Read the model definition and answer for the solid it produces. Units are mm, in the model's axes. Face numbers are marked on the shaded views. A direction names the side the tool comes from. Coordinates: 2 decimals unless noted, no trailing zeros. Loops run counter-clockwise (first coordinate to the right, second up) from the corner with the lowest first, then second, coordinate; pieces in that order, holes last.
Q1. The mould has two halves that part along Z. Classify the marked faces 4, 5 and 6: pulls with the +Z half, pulls with the -Z half, needs draft (parallel to the pull), parting line crosses it, or undercut.
Q2. Which of the six approach directions +Z, -Z, +X, -X, +Y, -Y give full straight-line access (tool end or side, diameter ignored) to the marked faces 1, 2 and 3?
Q3. Flat-ended cylindrical pins translate along their axes: P1, Ø12.5, axis at x = 92, y = 260, coming from the -Z side; P2, Ø1.5, axis at x = -83, y = 126.5, coming from the -Z side; P3, Ø12.5, axis at x = -92, y = 127.5, coming from the +Z side. Find the tip coordinate at first contact, or state that the pin passes through.
Q4. Section B-B (x = 92) is taken. Count the separate pieces of the cut face and the enclosed holes in it, then the cut area to 3 significant figures.
Q5. Straight lines are drawn through the part: line 1 (X direction, y = 127, z = 3); line 2 (Y direction, x = 92, z = 1); line 3 (Z direction, x = 95.5, y = -28). For each, find the intervals that lie inside material, in ascending order.
Q6. Section A-A (y = 127.5) is taken. Give the vertices of the cut face in (x, z), then the cut area to 3 significant figures.
Q7. Section C-C (y = -160) is taken. Give the vertices of the cut face in (x, z).
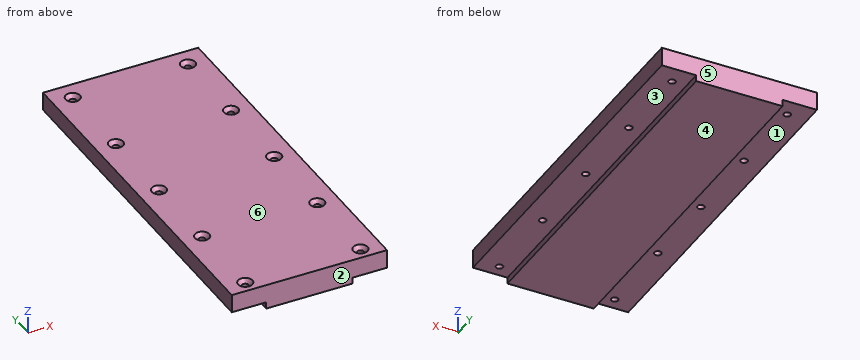
from build123d import *

# Parameters (mm, degrees)
SKETCH2_W                  = 580
SKETCH2_H                  = 248
BOSS_EXTRUDE1_DEPTH        = 20
SKETCH3_W                  = 55
SKETCH3_H                  = 10.706810323
SKETCH3_H_2                = 10
CUT_EXTRUDE1_DEPTH         = 594.444184402
F_11_0_11_DIAMETER_HOLE1_D = 11
LPATTERN1_COUNT            = 5
LPATTERN1_PITCH            = 132.5
CHAMFER1_SIZE              = 6


with BuildPart() as part:
    # Sketch2 → Boss-Extrude1 (new, symmetric)
    with BuildSketch(Plane(origin=(0, 0, 0), x_dir=(0, 1, 0), z_dir=(0, 0, 1))):
        Rectangle(SKETCH2_W, SKETCH2_H)
    extrude(amount=BOSS_EXTRUDE1_DEPTH, both=True)

    # Sketch3 → Cut-Extrude1 (cut, through all)
    with BuildSketch(Plane(origin=(0, 290, 0), x_dir=(-1, 0, 0), z_dir=(0, 1, 0))):
        with Locations((96.5, -14.646594839)):
            Rectangle(SKETCH3_W, SKETCH3_H)
        with Locations((-96.5, -15)):
            Rectangle(SKETCH3_W, SKETCH3_H_2)
    extrude(amount=-CUT_EXTRUDE1_DEPTH, mode=Mode.SUBTRACT)

    # Ø11.0 (11) Diameter Hole1 (through all)
    with Locations(Plane(origin=(-92, -270, 20), x_dir=(1, 0, 0), z_dir=(0, 0, 1))):
        with Locations((0, 0), (184, 0)):
            f_11_0_11_diameter_hole1 = Hole(F_11_0_11_DIAMETER_HOLE1_D / 2)

    # LPattern1: Ø11.0 (11) Diameter Hole1 ×5
    with Locations(*[(0, i * LPATTERN1_PITCH, 0) for i in range(1, LPATTERN1_COUNT)]):
        add(f_11_0_11_diameter_hole1, mode=Mode.SUBTRACT)

    # Chamfer1
    chamfer1_edges = [part.edges().sort_by_distance(p)[0] for p in [
        (97.5, -270, 20),
        (-86.5, -270, 20),
        (97.5, -137.5, 20),
        (-86.5, -137.5, 20),
        (97.5, -5, 20),
        (-86.5, -5, 20),
        (97.5, 127.5, 20),
        (-86.5, 127.5, 20),
        (97.5, 260, 20),
        (-86.5, 260, 20),
    ]]
    chamfer(chamfer1_edges, length=CHAMFER1_SIZE)


solid = part.part
Numbers:
1. face 4: pulls with the -Z half
1. face 5: needs draft
1. face 6: pulls with the +Z half
2. face 1: -Z, -X, +Y, -Y
2. face 2: +Z, -Z, +X, -X, -Y
2. face 3: -Z, +X, +Y, -Y
3. P1: stops at z = -10
3. P2: stops at z = -9.29
3. P3: stops at z = 14.75
4. separate pieces: 6
4. enclosed holes: 0
4. area: 15,600 mm2
5. line 1: x = -124 to -97.48, -86.52 to 86.52, 97.48 to 124
5. line 2: y = -290 to -275.5, -264.5 to -143, -132 to -10.5, 0.5 to 122, 133 to 254.5, 265.5 to 290
5. line 3: z = -10 to 20
6. outline: (-124, -9.29) - (-97.5, -9.29) - (-97.5, 14) - (-103.5, 20) - (-124, 20) - close; (-86.5, -9.29) - (-69, -9.29) - (-69, -20) - (69, -20) - (69, -10) - (86.5, -10) - (86.5, 14) - (80.5, 20) - (-80.5, 20) - (-86.5, 14) - close; (97.5, -10) - (124, -10) - (124, 20) - (103.5, 20) - (97.5, 14) - close
6. area: 8,060 mm2
7. outline: (-124, -9.29) - (-69, -9.29) - (-69, -20) - (69, -20) - (69, -10) - (124, -10) - (124, 20) - (-124, 20) - close
